Check sheet for the modelled part. Datum: model origin and axes. Units: mm. A direction names the side the tool comes from. Give positions to 0.01 mm unless a question says otherwise; leave off trailing zeros. Loops run counter-clockwise (first coordinate to the right, second up) from the corner with the lowest first, then second, coordinate; pieces in that order, holes last. Notation, with made-up numbers: (55, -31.75) - (63, -31.75) arc R29 ccw to (63, 2.25) - close; hole circle Ø3 at (18.25, 76.5). An arc over 180 degrees is marked (long way). Use one line per item in the form item = value.
from build123d import *

# Parameters (mm, degrees)
SWEEP2_PROFILE_R = 37.5
MOVE_FACE1_BY    = 100
MOVE_FACE2_BY    = 120


with BuildPart() as part:
    # Sweep2: sweep along a path in Sketch1
    with BuildLine(Plane.XY) as sweep2_path:
        Line((120, 0), (0, 0))
        Line((0, 0), (0, 300))
    # Sweep2 profile (on start of the path) → Sweep2 (sweep)
    with BuildSketch(Plane(origin=(120, 0, 0), x_dir=(0, -1, 0), z_dir=(-1, 0, 0))):
        Circle(SWEEP2_PROFILE_R)
    sweep(path=sweep2_path.line, transition=Transition.RIGHT)

    # Move Face1: a face moved outward by 100.0
    extrude(part.faces().sort_by_distance((0, 300, 0))[0], amount=MOVE_FACE1_BY, dir=(0, 1, 0))

    # Move Face2: a face moved outward by 120.0
    extrude(part.faces().sort_by_distance((0, 400, 0))[0], amount=MOVE_FACE2_BY, dir=(0, 1, 0))


solid = part.part
Item 1: Section check B-B on x = 65. Record the boundary of the cut face in (y, z).
Answer block:
outline = circle Ø75 at (0, 0)
Item 2: Section check A-A on z = 0. Record the boundary of the cut face in (x, y), then the cut area to 3 significant figures.
Answer block:
outline = (-37.5, -37.5) - (120, -37.5) - (120, 37.5) - (37.5, 37.5) - (37.5, 520) - (-37.5, 520) - close
area = 48,000 mm2
Item 3: Gauge pin test, flat ends, axial feed: P1, Ø1, axis at y = 310, z = -18.5, coming from the +X side; P2, Ø3, axis at x = 28, z = -13, coming from the -Y side; P3, Ø6, axis at x = 67, z = 18.5, coming from the -Y side; P4, Ø3, axis at y = 375, z = 0.5, coming from the -X side. Record the tip position at first contact, or that the pin passes through.
Answer block:
P1 = 32.9
P2 = -35.69
P3 = -34.15
P4 = -37.5
Item 4: Thickness scan on L1, parallel to X at y = 114.5, z = 0; L2, parallel to X at y = 49, z = 11; L3, parallel to Y at x = 97, z = 22.5. Record the ranges inside material, lowest first.
Answer block:
L1 = -37.5 to 37.5
L2 = -35.85 to 35.85
L3 = -30 to 30
Item 5: Section check C-C on y = 0. Record the boundary of the cut face in (x, z), then the cut area to 3 significant figures.
Answer block:
outline = (0, -37.5) - (120, -37.5) - (120, 37.5) - (0, 37.5) arc R37.5 ccw to start
area = 11,200 mm2
Item 6: Access from +Z, -Z, +X, -X, +Y, -Y to the whole of each face (thin tool, end or side, straight path). Record for faces 1 (the face through (57.65, -35.77, 11.26)), 2 (the face through (120, -1, 1)), 3 (the face through (-35.77, 237.35, 11.26)).
Answer block:
face_1 = +X
face_2 = +Z, -Z, +X, +Y, -Y
face_3 = +Y
